```python
from build123d import *

# Parameters (mm, degrees)
SKETCH_1_W          = 28
SKETCH_1_H          = 21.4
SKETCH_1_R          = 1.5
EXTRUDE_1_DEPTH     = 10
SKETCH_1_17_R       = 2.25
CUT_EXTRUDE_5_DEPTH = 8
CUT_EXTRUDE_START   = 14
SKETCH_2_R          = 0.85
CUT_EXTRUDE_1_DEPTH = 4
CUT_EXTRUDE_START_2 = -10
SKETCH_2_2_R        = 0.85
CUT_EXTRUDE_2_DEPTH = 4
CUT_EXTRUDE_START_3 = 13.9
SKETCH_3_R          = 0.85
CUT_EXTRUDE_3_DEPTH = 4
CUT_EXTRUDE_START_4 = -3.5
SKETCH_3_2_R        = 0.85
CUT_EXTRUDE_4_DEPTH = 4


with BuildPart() as part:
    # 草图1 → 凸台-拉伸1 (new body)
    with BuildSketch(Plane(origin=(0, 0, 0), x_dir=(1, 0, 0), z_dir=(0, 1, 0))):
        with Locations((0, -3.2)):
            Rectangle(SKETCH_1_W, SKETCH_1_H)
        with Locations(Location((-8, 0, 0), (0, 0, 270))):
            Circle(SKETCH_1_R, mode=Mode.SUBTRACT)
        with BuildLine():
            ThreePointArc((5.5, 0), (0, -5.5), (-5.5, 0))
            ThreePointArc((-5.5, 0), (0, 5.5), (5.5, 0))
        make_face(mode=Mode.SUBTRACT)
        with Locations(Location((8, 0, 0), (0, 0, 270))):
            Circle(SKETCH_1_R, mode=Mode.SUBTRACT)
        with Locations(Location((0, -10.9, 0), (0, 0, 270))):
            Circle(SKETCH_1_R, mode=Mode.SUBTRACT)
    extrude(amount=EXTRUDE_1_DEPTH)

    # 草图1<17> → 切除-拉伸5 (cut)
    with BuildSketch(Plane(origin=(0, 0, 0), x_dir=(1, 0, 0), z_dir=(0, 1, 0))):
        with Locations(Location((-8, 0, 0), (0, 0, 270))):
            Circle(SKETCH_1_17_R)
        with Locations(Location((8, 0, 0), (0, 0, 270))):
            Circle(SKETCH_1_17_R)
    extrude(amount=CUT_EXTRUDE_5_DEPTH, mode=Mode.SUBTRACT)

    # 草图2 → 切除-拉伸1 (cut)
    with BuildSketch(Plane(origin=(0, 0, 0), x_dir=(0, 0, -1), z_dir=(1, 0, 0)).offset(CUT_EXTRUDE_START)):
        with Locations(Location((-8.9, 5, 0), (0, 0, 180))):
            Circle(SKETCH_2_R)
        with Locations(Location((2.5, 5, 0), (0, 0, 180))):
            Circle(SKETCH_2_R)
    extrude(amount=-CUT_EXTRUDE_1_DEPTH, mode=Mode.SUBTRACT)

    # 草图2<2> → 切除-拉伸2 (cut)
    with BuildSketch(Plane(origin=(0, 0, 0), x_dir=(0, 0, -1), z_dir=(1, 0, 0)).offset(CUT_EXTRUDE_START_2)):
        with Locations(Location((-8.9, 5, 0), (0, 0, 180))):
            Circle(SKETCH_2_2_R)
        with Locations(Location((2.5, 5, 0), (0, 0, 180))):
            Circle(SKETCH_2_2_R)
    extrude(amount=-CUT_EXTRUDE_2_DEPTH, mode=Mode.SUBTRACT)

    # 草图3 → 切除-拉伸3 (cut)
    with BuildSketch(Plane.XY.offset(CUT_EXTRUDE_START_3)):
        with Locations((-9, 5)):
            Circle(SKETCH_3_R)
        with Locations((9, 5)):
            Circle(SKETCH_3_R)
    extrude(amount=-CUT_EXTRUDE_3_DEPTH, mode=Mode.SUBTRACT)

    # 草图3<2> → 切除-拉伸4 (cut)
    with BuildSketch(Plane.XY.offset(CUT_EXTRUDE_START_4)):
        with Locations((-9, 5)):
            Circle(SKETCH_3_2_R)
        with Locations((9, 5)):
            Circle(SKETCH_3_2_R)
    extrude(amount=-CUT_EXTRUDE_4_DEPTH, mode=Mode.SUBTRACT)


solid = part.part
```
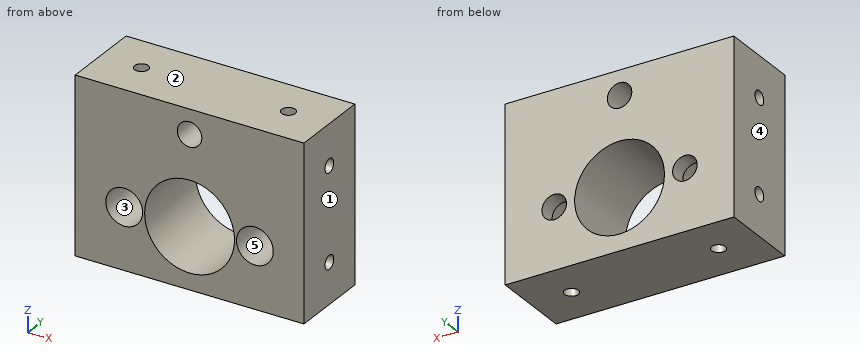
Geometry: final body of the model. Coordinates: model frame, mm. Face numbers are marked on the shaded views. A direction names the side the tool comes from. Coordinates: 2 decimals unless noted, no trailing zeros. Order: outer loops, then holes, each group sorted by start corner. A loop starts at its lowest first (then second) coordinate and runs counter-clockwise, first axis right, second up. Notation, with made-up numbers: (40.5, 31.25) - (93.5, 31.25) arc R16 ccw to (93.5, 47.25) - close; hole circle Ø3 at (79, 73). An arc over 180 degrees is marked (long way). Write each question's results on one line, items separated by ' | '.
(1) Section query C-C, the plane y = 7. Return the cut outline in (x, z).
Values found:
outline: (-14, -7.5) - (14, -7.5) - (14, 13.9) - (-14, 13.9) - close; hole circle Ø4.5 at (-8, 0); hole circle Ø11 at (0, 0); hole circle Ø3 at (0, 10.9); hole circle Ø4.5 at (8, 0)
(2) Section query B-B, the plane x = 0. Return the cut outline in (y, z), plus the area to 3 significant figures.
Values found:
outline: (0, -7.5) - (10, -7.5) - (10, -5.5) - (0, -5.5) - close; (0, 5.5) - (10, 5.5) - (10, 9.4) - (0, 9.4) - close; (0, 12.4) - (10, 12.4) - (10, 13.9) - (0, 13.9) - close | area: 74.0 mm²
(3) Line query: line 1 (X direction, y = 6, z = 0); line 2 (Z direction, x = 10.9, y = 5); line 3 (Z direction, x = 8, y = 8.75). Output: solid intervals per line, ascending. Write a range as [from, to].
Values found:
line 1: x = [-14, -10.25], [-5.75, -5.5], [5.5, 5.75], [10.25, 14] | line 2: z = [-7.5, -3.35], [-1.65, 8.05], [9.75, 13.9] | line 3: z = [-7.5, -1.5], [1.5, 13.9]
(4) Mould query, pull axis X, two halves, no side actions, for the marked faces 1, 2 and 3. Classes: +X half, -X half, draft (parallel to the pull), parting line (faces both ways), or undercut.
Values found:
face 1: +X half | face 2: draft | face 3: undercut
(5) First-contact query: pin 1 Ø1.4 at (y, z) = (5, -2.5) entering from +X; pin 2 Ø1.4 at (x, y) = (-9, 5) entering from +Z. Flat tips, straight axial feed; report the tip coordinate or a pass-through.
Values found:
pin 1: stops at x = 10 | pin 2: stops at z = 9.9
(6) Section query D-D, the plane x = 11.75. Return the cut outline in (y, z).
Values found:
outline: (0, -7.5) - (10, -7.5) - (10, 13.9) - (0, 13.9) - close; hole circle Ø1.7 at (5, -2.5); hole circle Ø1.7 at (5, 8.9)
(7) Section query A-A, the plane z = 10.9. Return the cut outline in (x, y), plus the area to 3 significant figures.
Values found:
outline: (-14, 0) - (-1.5, 0) - (-1.5, 10) - (-14, 10) - close; (1.5, 0) - (14, 0) - (14, 10) - (1.5, 10) - close; hole circle Ø1.7 at (-9, 5); hole circle Ø1.7 at (9, 5) | area: 245 mm²
(8) Set-up query: the marked faces 4 and 5. Return all of +Z, -Z, +X, -X, +Y, -Y with unobstructed straight access to the full face (end or side cutting, diameter ignored); none if empty.
Values found:
face 4: +Z, -Z, -X, +Y, -Y | face 5: -Y
